from build123d import *

# Parameters (mm, degrees)
ESBO_O1_R                = 17.075
RESSALTO_EXTRUS_O1_DEPTH = 38.3
ESBO_O2_R                = 8.85
RESSALTO_EXTRUS_O2_DEPTH = 5
ESBO_O3_R                = 4
RESSALTO_EXTRUS_O3_DEPTH = 3
ESBO_O5_R                = 1
RESSALTO_EXTRUS_O4_DEPTH = 7
ESBO_O6_R                = 3
RESSALTO_EXTRUS_O5_DEPTH = 4


with BuildPart() as part:
    # Esboço1 → Ressalto-extrusão1 (new body)
    with BuildSketch(Plane(origin=(0, 0, 0), x_dir=(1, 0, 0), z_dir=(0, 1, 0))):
        with Locations(Location((0, 0, 0), (0, 0, 270))):
            Circle(ESBO_O1_R)
    extrude(amount=RESSALTO_EXTRUS_O1_DEPTH)

    # Esboço2 → Ressalto-extrusão2 (add)
    with BuildSketch(Plane(origin=(0, 38.3, 0), x_dir=(1, 0, 0), z_dir=(0, 1, 0))):
        with Locations(Location((0, 0, 0), (0, 0, 270))):
            Circle(ESBO_O2_R)
    extrude(amount=RESSALTO_EXTRUS_O2_DEPTH)

    # Esboço3 → Ressalto-extrusão3 (add)
    with BuildSketch(Plane.XZ):
        with Locations(Location((0, 0, 0), (0, 0, 270))):
            Circle(ESBO_O3_R)
    extrude(amount=RESSALTO_EXTRUS_O3_DEPTH)

    # Esboço5 → Ressalto-extrusão4 (add)
    with BuildSketch(Plane.XZ.offset(3)):
        with Locations(Location((0, 0, 0), (0, 0, 270))):
            Circle(ESBO_O5_R)
    extrude(amount=RESSALTO_EXTRUS_O4_DEPTH)

    # Esboço6 → Ressalto-extrusão5 (add)
    with BuildSketch(Plane.XZ.offset(10)):
        with Locations(Location((0, 0, 0), (0, 0, 270))):
            Circle(ESBO_O6_R)
    extrude(amount=-RESSALTO_EXTRUS_O5_DEPTH)


solid = part.part
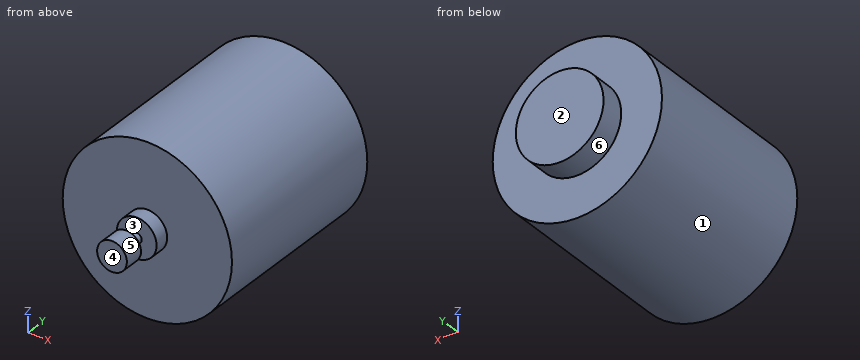
Verification items for the finished model (mm, model axes). Face numbers are marked on the shaded views. A direction names the side the tool comes from. Give positions to 0.01 mm unless a question says otherwise; leave off trailing zeros. Loops run counter-clockwise (first coordinate to the right, second up) from the corner with the lowest first, then second, coordinate; pieces in that order, holes last. Notation, with made-up numbers: (41.25, 28) - (93.25, 28) arc R8 cw to (93.25, 40) - close; hole circle Ø10 at (-4, 61). An arc over 180 degrees is marked (long way). Write item = value, one per line. Start each with the question number.
Q1. Cross-section at A-A, the plane z = 0. Enter the section's corners in (x, y) (3 decimals).
Q2. Cross-section at B-B, the plane x = 0. Enter the section's corners in (y, z) (3 decimals).
Q3. Depth check by flat-ended pin: P1, Ø4, axis at x = -12.5, y = 13, coming from the +Z side (3 decimals); P2, Ø8, axis at x = 4.5, y = 4, coming from the +Z side; P3, Ø2, axis at y = 13.5, z = 5, coming from the -X side. Enter the tip coordinate at first touch or a pass-through.
Q4. Cross-section at C-C, the plane y = 40. Enter the section's corners in (x, z).
Q5. Thickness scan on line 1 (Y direction, x = 2.5, z = 11); line 2 (Y direction, x = 4, z = -6); line 3 (Z direction, x = 1.5, y = 38). Record the ranges inside material, lowest first.
Q6. Mould release check, pull along Y, two halves, no side actions. Record for the marked faces 1, 2 and 3: released by +Y, released by -Y, zero draft, split by the parting line, or undercut.
Q7. Tool access check on the marked faces 4, 5 and 6. Record the directions out of +Z, -Z, +X, -X, +Y, -Y that give a thin tool (end or side, any length) a straight path to the whole face; none if there is none.
Q8. Cross-section at D-D, the plane x = 6. Enter the section's corners in (y, z).
Answer key:
q1.outline = (-17.075, 0) - (-4, 0) - (-4, -3) - (-1, -3) - (-1, -6) - (-3, -6) - (-3, -10) - (3, -10) - (3, -6) - (1, -6) - (1, -3) - (4, -3) - (4, 0) - (17.075, 0) - (17.075, 38.3) - (8.85, 38.3) - (8.85, 43.3) - (-8.85, 43.3) - (-8.85, 38.3) - (-17.075, 38.3) - close
q2.outline = (-10, -3) - (-6, -3) - (-6, -1) - (-3, -1) - (-3, -4) - (0, -4) - (0, -17.075) - (38.3, -17.075) - (38.3, -8.85) - (43.3, -8.85) - (43.3, 8.85) - (38.3, 8.85) - (38.3, 17.075) - (0, 17.075) - (0, 4) - (-3, 4) - (-3, 1) - (-6, 1) - (-6, 3) - (-10, 3) - close
q3.P1 = 13.465
q3.P2 = 17.07
q3.P3 = -16.6
q4.outline = circle Ø17.7 at (0, 0)
q5.line_1 = 0 to 38.3
q5.line_2 = 0 to 43.3
q5.line_3 = -17.01 to 17.01
q6.face_1 = zero draft
q6.face_2 = released by +Y
q6.face_3 = undercut
q7.face_4 = +Z, -Z, +X, -X, -Y
q7.face_5 = -Y
q7.face_6 = +Y
q8.outline = (0, -15.99) - (38.3, -15.99) - (38.3, -6.51) - (43.3, -6.51) - (43.3, 6.51) - (38.3, 6.51) - (38.3, 15.99) - (0, 15.99) - close
